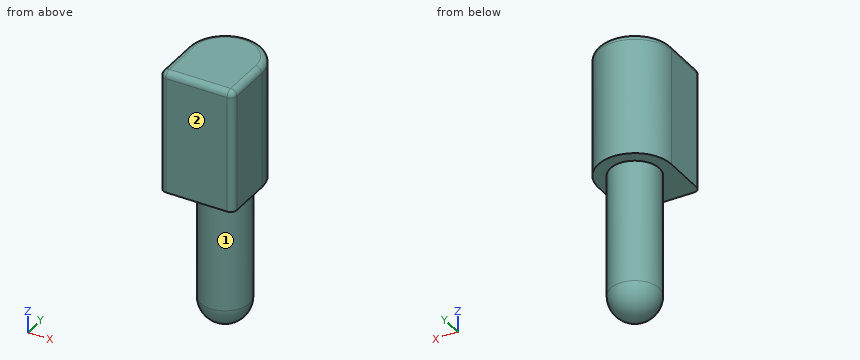
from build123d import *

# Parameters (mm, degrees)
F1_DEPTH = 25
F2_R     = 1.25
F3_R     = 5
F4_DEPTH = 30
F5_R     = 5


with BuildPart() as f1:
    # F0 (on Top) → F1 (new body)
    with BuildSketch(Plane.XY):
        with BuildLine():
            Line((-7.5, 0), (-7.5, -10))
            Line((-7.5, -10), (7.5, -10))
            Line((7.5, -10), (7.5, 0))
            ThreePointArc((7.5, 0), (0, 7.5), (-7.5, 0))
        make_face()
    extrude(amount=F1_DEPTH)

    # F2
    f2_edges = [f1.edges().sort_by_distance(p)[0] for p in [
        (7.5, -10, 12.5),
        (0, -10, 25),
        (7.5, -5, 25),
        (-7.5, -10, 12.5),
    ]]
    fillet(f2_edges, radius=F2_R)

    # F3 (on face) → F4 (join)
    with BuildSketch(Plane(origin=(0, 0, 0), x_dir=(1, 0, 0), z_dir=(0, 0, -1))):
        Circle(F3_R)
    extrude(amount=F4_DEPTH)

    # F5
    f5_edges = [f1.edges().sort_by_distance(p)[0] for p in [
        (-5, 0, -30),
    ]]
    fillet(f5_edges, radius=F5_R)


solid = f1.part
Build history of the part. All positions in model axes, mm. Face numbers are marked on the shaded views. A direction names the side the tool comes from. Give positions to 0.01 mm unless a question says otherwise; leave off trailing zeros. Write each loop counter-clockwise with the first axis right and the second up, starting at its lowest first coordinate (ties: lowest second). Pieces come first, ordered by that corner, then holes. Notation, with made-up numbers: (-9, -33) - (19, -33) arc R35 ccw to (19, -1) - close; hole circle Ø11 at (24, 80.5). An arc over 180 degrees is marked (long way). Use one line per item in the form item = value. Start each with the question number.
1. Drop flat-ended pins along their axis: pin 1 Ø3 at (y, z) = (-3.5, -18) entering from +X; pin 2 Ø7.5 at (x, y) = (0.5, 2.5) entering from -Z; pin 3 Ø6 at (x, z) = (5, -15) entering from +Y; pin 4 Ø2 at (y, z) = (-5, -21) entering from -X. Give the stop position or say it passes through.
2. Band-saw the part on C-C on y = -1. Write the cut outline in (x, z), plus the area to 3 significant figures.
3. Band-saw the part on A-A on x = 0. Write the cut outline in (y, z).
4. Band-saw the part on D-D on z = -16. Write the cut outline in (x, y).
5. Probe line 1 (Y direction, x = 0.25, z = 22); line 2 (Z direction, x = 4.5, y = -4.5); line 3 (X direction, y = 0.25, z = -20). List the from-to ranges inside material, lowest first. Write a range as [from, to].
6. Band-saw the part on B-B on z = 10. Write the cut outline in (x, y), plus the area to 3 significant figures.
7. 3-axis set-ups, long thin cutter, end or side, ignore diameter. For the marked faces 1 and 2: which of +Z, -Z, +X, -X, +Y, -Y reach the whole face in a straight line?
Conclusion:
q1.pin_1 = 4.58
q1.pin_2 = -30
q1.pin_3 = 4.58
q1.pin_4 = -3
q2.outline = (-7.5, 0) - (-4.9, 0) - (-4.9, -25) arc R4.9 ccw to (4.9, -25) - (4.9, 0) - (7.5, 0) - (7.5, 23.75) arc R1.25 ccw to (6.25, 25) - (-6.25, 25) arc R1.25 ccw to (-7.5, 23.75) - close
q2.area = 657 mm²
q3.outline = (-10, 0) - (-5, 0) - (-5, -25) arc R5 ccw to (5, -25) - (5, 0) - (7.5, 0) - (7.5, 23.75) arc R1.25 ccw to (6.25, 25) - (-8.75, 25) arc R1.25 ccw to (-10, 23.75) - close
q4.outline = circle Ø10 at (0, 0)
q5.line_1 = [-10, 7.5]
q5.line_2 = [0, 25]
q5.line_3 = [-4.99, 4.99]
q6.outline = (-7.5, -8.75) arc R1.25 ccw to (-6.25, -10) - (6.25, -10) arc R1.25 ccw to (7.5, -8.75) - (7.5, 0) arc R7.5 ccw to (-7.5, 0) - close
q6.area = 238 mm²
q7.face_1 = -Z
q7.face_2 = +Z, -Z, +X, -X, -Y
